CAD build for the part. Positions are in the model's coordinates, mm. A direction names the side the tool comes from. Coordinates: 2 decimals unless noted, no trailing zeros. Loops run counter-clockwise (first coordinate to the right, second up) from the corner with the lowest first, then second, coordinate; pieces in that order, holes last.
1) Which spindle directions (+Z, -Z, +X, -X, +Y, -Y) get a long thin tool onto all of the face, cutting with end or side? Do faces 4 (the flat face through (97, -50.8, 2)), 5 (the flat face through (48, -25, 3.175)). Say none if no direction does.
2) Wall check: line 1 along Z through (x, y) = (142, -16) (3 decimals); line 2 along Z through (x, y) = (144, -14). Give the ranges that are in metal, low to high.
3) Saw through at B-B, the plane x = 80.5. Write the cut outline in (y, z) (3 decimals), and give its area (3 significant figures).
4) Saw through at A-A, the plane y = -36. Write the cut outline in (x, z) (1 decimal).
5) Pin check, flat tips, straight feed: pin 1 Ø10 at (x, y) = (79, -14) entering from +Z; pin 2 Ø16 at (x, y) = (49, -16.5) entering from +Z; pin 3 Ø5 at (x, y) = (124, -28.5) entering from +Z (3 decimals). Stop position of each tip, or through.
6) Two-plate mould, pull along X, no slides. Class faces 1 (the flat face through (97, 0, 2)), 2 (the flat face through (12.7, -25, 2)), 3 (the cylindrical face through (38.821, -25.044, 4.762)): +X half, -X half, draft (parallel to the pull), parting line (faces both ways), or undercut.
```python
from build123d import *

# Parameters (mm, degrees)
F1_DEPTH = 50.8


with BuildPart() as f1:
    # F0 (on Front) → F1 (new body)
    with BuildSketch(Plane.XZ):
        with BuildLine():
            Line((12.7, 3.175), (12.7, 0))
            Line((12.7, 0), (182.88, 0))
            Line((182.88, 0), (182.88, 3.175))
            Line((182.88, 3.175), (179.3875, 3.175))
            ThreePointArc((179.3875, 3.175), (177.8, 4.7625), (176.2125, 3.175))
            Line((176.2125, 3.175), (168.8211, 3.175))
            ThreePointArc((168.8211, 3.175), (167.2336, 4.7625), (165.6461, 3.175))
            Line((165.6461, 3.175), (157.6197, 3.175))
            ThreePointArc((157.6197, 3.175), (156.0322, 4.7625), (154.4447, 3.175))
            Line((154.4447, 3.175), (145.2499, 3.175))
            ThreePointArc((145.2499, 3.175), (143.6624, 4.7625), (142.0749, 3.175))
            Line((142.0749, 3.175), (133.1849, 3.175))
            ThreePointArc((133.1849, 3.175), (131.5974, 4.7625), (130.0099, 3.175))
            Line((130.0099, 3.175), (119.8499, 3.175))
            ThreePointArc((119.8499, 3.175), (118.2624, 4.7625), (116.6749, 3.175))
            Line((116.6749, 3.175), (105.7529, 3.175))
            ThreePointArc((105.7529, 3.175), (104.1654, 4.7625), (102.5779, 3.175))
            Line((102.5779, 3.175), (90.7923, 3.175))
            ThreePointArc((90.7923, 3.175), (89.2048, 4.7625), (87.6173, 3.175))
            Line((87.6173, 3.175), (74.9427, 3.175))
            ThreePointArc((74.9427, 3.175), (73.3552, 4.7625), (71.7677, 3.175))
            Line((71.7677, 3.175), (58.1533, 3.175))
            ThreePointArc((58.1533, 3.175), (56.5658, 4.7625), (54.9783, 3.175))
            Line((54.9783, 3.175), (40.3733, 3.175))
            ThreePointArc((40.3733, 3.175), (38.7858, 4.7625), (37.1983, 3.175))
            Line((37.1983, 3.175), (21.5519, 3.175))
            ThreePointArc((21.5519, 3.175), (19.9644, 4.7625), (18.3769, 3.175))
            Line((18.3769, 3.175), (12.7, 3.175))
        make_face()
    extrude(amount=F1_DEPTH)


solid = f1.part
```
Data:
1. face 4: +Z, -Z, +X, -X, -Y
1. face 5: +Z, +Y, -Y
2. line 1: z = 0 to 3.175
2. line 2: z = 0 to 4.73
3. outline: (-50.8, 0) - (0, 0) - (0, 3.175) - (-50.8, 3.175) - close
3. area: 161 mm2
4. outline: (12.7, 0) - (182.9, 0) - (182.9, 3.2) - (179.4, 3.2) arc R1.6 ccw to (176.2, 3.2) - (168.8, 3.2) arc R1.6 ccw to (165.6, 3.2) - (157.6, 3.2) arc R1.6 ccw to (154.4, 3.2) - (145.2, 3.2) arc R1.6 ccw to (142.1, 3.2) - (133.2, 3.2) arc R1.6 ccw to (130, 3.2) - (119.8, 3.2) arc R1.6 ccw to (116.7, 3.2) - (105.8, 3.2) arc R1.6 ccw to (102.6, 3.2) - (90.8, 3.2) arc R1.6 ccw to (87.6, 3.2) - (74.9, 3.2) arc R1.6 ccw to (71.8, 3.2) - (58.2, 3.2) arc R1.6 ccw to (55, 3.2) - (40.4, 3.2) arc R1.6 ccw to (37.2, 3.2) - (21.6, 3.2) arc R1.6 ccw to (18.4, 3.2) - (12.7, 3.2) - close
5. pin 1: stops at z = 4.63
5. pin 2: stops at z = 4.76
5. pin 3: stops at z = 3.175
6. face 1: draft
6. face 2: -X half
6. face 3: undercut
